Study the drawing (mm; zero at the part's minimum x, y, z) and answer. A direction names the side the tool comes from. Give positions to 0.01 mm unless a question says otherwise; leave off trailing zeros. Write each loop counter-clockwise with the first axis right and the second up, starting at its lowest first coordinate (ties: lowest second). Pieces come first, ordered by that corner, then holes. Notation, with made-up numbers: (8.25, 74) -> (45.25, 74) arc R16 cw to (45.25, 80) -> close; hole circle Ø8 at (13.25, 6). An arc over 180 degrees is marked (long way). Put each result on its own line as item: value. Start each with the question number.
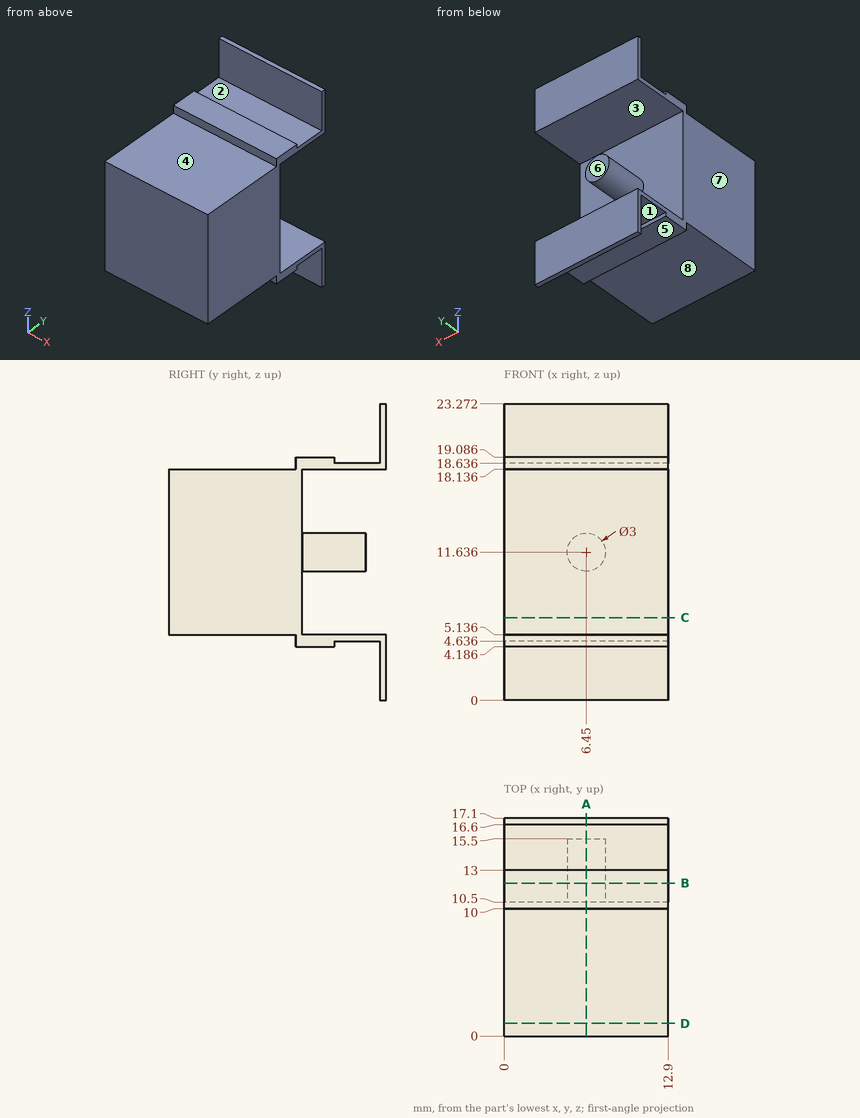
1) A cutting plane is placed at D-D on y = 1. Give the vertices of the cut face in (x, z).
2) A cutting plane is placed at C-C on z = 6.5. Give the vertices of the cut face in (x, y), and give its area (3 significant figures).
3) For a pull along Z with two mould halves and no side action, classify the marked faces 6, 7 and 8 as pulls with the +Z half, pulls with the -Z half, needs draft (parallel to the pull), parting line crosses it, or undercut.
4) Straight lines are drawn through the part: line 1 (Z direction, x = 4.25, y = 12); line 2 (Z direction, x = 12, y = 16.5); line 3 (Y direction, x = 2.5, z = 6.25). For each, find the intervals that lie inside material, in ascending order. Write a range as [from, to].
5) Each of these flat-tipped pins is pushed along its axis until it touches: pin 1 Ø2 at (x, y) = (5.5, 8.5) entering from -Z; pin 2 Ø3.5 at (x, z) = (6.5, 11.5) entering from +Y; pin 3 Ø2 at (x, z) = (10.5, 14) entering from +Y. Where does it stop, or does it pass through?
6) For the marked faces 1, 2, 3, 4 and 5, determine the directions among +Z, -Z, +X, -X, +Y, -Y from which every point of the face is accessible in a straight line to the end or side of a thin tool.
7) A cutting plane is placed at A-A on x = 6.45. Give the vertices of the cut face in (y, z), and give its area (3 significant figures).
8) A cutting plane is placed at B-B on y = 12. Give the vertices of the cut face in (x, z).
Results found:
1. outline: (0, 5.14) -> (12.9, 5.14) -> (12.9, 18.14) -> (0, 18.14) -> close
2. outline: (0, 0) -> (12.9, 0) -> (12.9, 10.5) -> (0, 10.5) -> close
2. area: 135 mm²
3. face 6: undercut
3. face 7: needs draft
3. face 8: pulls with the -Z half
4. line 1: z = [4.19, 5.14], [18.14, 19.09]
4. line 2: z = [4.64, 5.14], [18.14, 18.64]
4. line 3: y = [0, 10.5]
5. pin 1: stops at z = 5.14
5. pin 2: stops at y = 15.5
5. pin 3: stops at y = 10.5
6. face 1: -Z, +X, -X
6. face 2: +Z, +X, -X
6. face 3: +X, -X, +Y
6. face 4: +Z, +X, -X, -Y
6. face 5: -Z, +X, -X, -Y
7. outline: (0, 5.14) -> (10, 5.14) -> (10, 4.19) -> (13, 4.19) -> (13, 4.64) -> (16.6, 4.64) -> (16.6, 0) -> (17.1, 0) -> (17.1, 5.14) -> (10.5, 5.14) -> (10.5, 10.14) -> (15.5, 10.14) -> (15.5, 13.14) -> (10.5, 13.14) -> (10.5, 18.14) -> (17.1, 18.14) -> (17.1, 23.27) -> (16.6, 23.27) -> (16.6, 18.64) -> (13, 18.64) -> (13, 19.09) -> (10, 19.09) -> (10, 18.14) -> (0, 18.14) -> close
7. area: 166 mm²
8. outline: (0, 4.19) -> (12.9, 4.19) -> (12.9, 5.14) -> (0, 5.14) -> close; (0, 18.14) -> (12.9, 18.14) -> (12.9, 19.09) -> (0, 19.09) -> close; circle Ø3 at (6.45, 11.64)
